```python
from build123d import *

# Parameters (mm, degrees)
SKETCH023_R     = 30
SKETCH023_R_2   = 19
PAD007_DEPTH    = 2
SKETCH125_R     = 2
POCKET053_DEPTH = 171.753761


with BuildPart() as part:
    # Sketch023 → Pad007 (new body)
    with BuildSketch(Plane.XY):
        Circle(SKETCH023_R)
        Circle(SKETCH023_R_2, mode=Mode.SUBTRACT)
    extrude(amount=PAD007_DEPTH)

    # Sketch125 → Pocket053 (cut, through all)
    with BuildSketch(Plane.XY.offset(2)):
        with Locations((-22.5, -5.2)):
            Circle(SKETCH125_R)
    pocket053 = extrude(amount=-POCKET053_DEPTH, mode=Mode.SUBTRACT)

    # Mirrored: Pocket053 across Sketch125 V_Axis
    add(pocket053.mirror(Plane(origin=(0, 0, 2), x_dir=(0, 0, 1), z_dir=(1, 0, 0))), mode=Mode.SUBTRACT)


with BuildPart() as part_1:
    # Body007 placement: moved
    add(part.part.moved(Location((0, 0, 64))))


solid = part_1.part
```
The model under review builds one solid part; all positions refer to its coordinate system, in mm. Give positions to 0.01 mm unless a question says otherwise; leave off trailing zeros. Order: outer loops, then holes, each group sorted by start corner. A loop starts at its lowest first (then second) coordinate and runs counter-clockwise, first axis right, second up. Notation, with made-up numbers: (36, 30.5) - (88, 30.5) arc R24 cw to (88, 57.5) - close; hole circle Ø5 at (-18.5, 55.25). An arc over 180 degrees is marked (long way). Use CSV: the item, a comma, the result in double quotes. Start each with the question number.
Q1. We need section A-A, the plane x = 0. Write out the cut boundary in (y, z).
Q2. We need section D-D, the plane x = -26. Write out the cut boundary in (y, z).
Q3. To check wall thickness, follow line 1 along Y through (x, z) = (0, 64.65); line 2 along X through (y, z) = (-13.5, 65.2); line 3 along Y through (x, z) = (-16.5, 65.85). State the ranges of each line that lie inside material, in increasing order. Write a range as [from, to].
Q4. We need section C-C, the plane z = 65.25. Write out the cut boundary in (x, y), and give its area (3 significant figures).
Q5. Clearance check with flat-ended pins moving along their axes: pin 1 Ø1 at (y, z) = (9, 64.5) entering from +X; pin 2 Ø1 at (x, z) = (14.5, 65) entering from -Y. State where each tip first meets the part, or that it passes through.
Outcome:
1,outline,"(-30, 64) - (-19, 64) - (-19, 66) - (-30, 66) - close; (19, 64) - (30, 64) - (30, 66) - (19, 66) - close"
2,outline,"(-14.97, 64) - (14.97, 64) - (14.97, 66) - (-14.97, 66) - close"
3,line 1,"y = [-30, -19], [19, 30]"
3,line 2,"x = [-26.79, -13.37], [13.37, 26.79]"
3,line 3,"y = [-25.05, -9.42], [9.42, 25.05]"
4,outline,"circle Ø60 at (0, 0); hole circle Ø4 at (-22.5, -5.2); hole circle Ø38 at (0, 0); hole circle Ø4 at (22.5, -5.2)"
4,area,"1,670 mm^2"
5,pin 1,"stops at x = 28.77"
5,pin 2,"stops at y = -26.53"
